Autodesk Inventor part; units mm, degrees
ref_plane "Work Plane1" through (2.75, 0, 0) normal (0, -1, 0) x (1, 0, 0)
ref_plane "YZ Plane" through (0, 0, 0) normal (1, 0, 0) x (0, 1, 0)
ref_plane "XZ Plane" through (0, 0, 0) normal (0, 1, 0) x (-1, 0, 0)
sketch "Skizze1" plane through (0, 0, 0) normal (0, 0, 1) x (1, 0, 0)
  line L0 (40, 4) -> (40, 0)
  line L1 (-12.8, 0) -> (40, 0)
  line L2 (-23.36, 0) -> (50.56, 0)
  line L3 (0, 4.8) -> (0, -0.8)
  line L4 (-12.8, 4) -> (-12.8, 0)
  line L5 (18, 4) -> (18, 0) construction
  line L6 (-23.36, 0) -> (50.56, 0)
  line L7 (-12.8, 4) -> (40, 4)
  dimension "d4" = 12.8
  dimension "d5" = 40
  dimension "d6" = 22
  dimension "d13" = 8
revolve "Körper" add sketch "Skizze1" angle 360 about axis through (-12.8, 0, 0) along (1, 0, 0)
thread "Gewinde1"
thread "Gewinde2"
chamfer "Fase1" distance 0.7678 distance2 1.25 1 edges at (40, -4, 0) measured on face at (40, -0.0467, 2.2623)
chamfer "Fase2" distance 0.7678 distance2 1.25 1 edges at (-12.8, -4, 0) measured on face at (21.5667, 3.987, -0.3219)
ref_plane "Work Plane1" through (2.75, 0, 0) normal (0, -1, 0) x (1, 0, 0)
equation "\"d4\" = KOH"
equation "\"d5\" = NLG"
equation "\"d6\" = GEL"
equation "\"d13\" = GD"
equation "\"d1\" = KOH"
equation "\"d7\" = GEL + GAL"
equation "\"d10\" = -0.5 * SPD + 0.5 * GD"
equation "\"d12\" = -0.5 * SPD + 0.5 * GD"
equation "\"NLG\" = 40"
equation "\"GEL\" = 22"
equation "\"GAL\" = 0.61345 * PTC"
equation "\"SPD\" = 5.5"
equation "\"d0\" = GD"
equation "\"GUL\" = 0.61345 * PTC"
equation "\"KOH\" = 12.8"
equation "\"GD\" = 8"
equation "\"BDM\" = NND"
equation "\"GUL1\" = GUL"
equation "\"GAL1\" = GAL"
equation "\"d80\" = -GUL - GEL"
equation "\"d86\" = -KOH + GUL1"
equation "\"PTC\" = 1.25"
equation "\"THREADDIA\" = 8"
equation "\"TOA\" = 30deg"
equation "\"NND\" = 8"
equation "\"GD1\" = THREADDIA - 1.2269 * PTC"
properties part number "DIN 835 - M8 x 40" material "Stahl, weich"
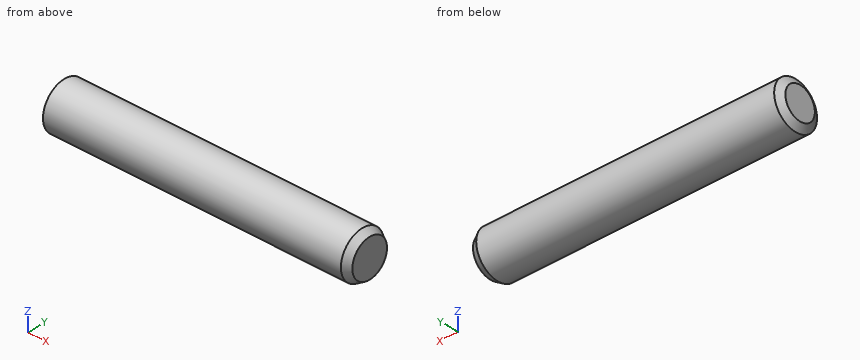
Check sheet for the modelled part. Datum: model origin and axes. Units: mm. Round coordinates to 2 decimals unless told otherwise and drop trailing zeros. Order: outer loops, then holes, each group sorted by start corner. A loop starts at its lowest first (then second) coordinate and runs counter-clockwise, first axis right, second up. Notation, with made-up numbers: M 10,60.25 L 39,60.25 A22 ccw 39,86.25 Z; hole C -13.75,47.5 d6. An arc over 180 degrees is marked long. Answer in a Markdown table with one row per item.
(1) Gauge pin test, flat end, axial feed: pin 1 (1.5 mm diameter, centred on x = 29, z = -3, fed in from -Y). Record the tip position at first contact, or that the pin passes through.
Findings:
| item | result |
|---|---|
| pin 1 | stops at y = -3.31 |
(2) Material ranges on line 1 along Z through (x, y) = (24, 0.25); line 2 along X through (y, z) = (-1.75, -2.75), recorded low to high. Write a range as from..to.
Findings:
| item | result |
|---|---|
| line 1 | z = -3.99..3.99 |
| line 2 | x = -12.49..39.96 |
(3) Section check A-A on x = 28. Record the boundary of the cut face in (y, z), plus the area to 3 significant figures.
Findings:
| item | result |
|---|---|
| outline | C 0,0 d8 |
| area | 50.3 mm^2 |
